from build123d import *

# Parameters (mm, degrees)
SKETCH1_R               = 14.287500000000001
BOSS_EXTRUDE1_DEPTH     = 165.1
CUT_EXTRUDE1_DEPTH      = 258.8795903614708
CUT_EXTRUDE1_DEPTH_BACK = 258.8795903614708
BOSS_EXTRUDE2_DEPTH     = 152.4
FILLET2_R               = 76.2


with BuildPart() as part:
    # Sketch1 → Boss-Extrude1 (new body)
    with BuildSketch(Plane.XY):
        with BuildLine():
            Line((6.759931115856893, 24.483940273347972), (-169.05197980207154, 73.02499999999999))
            ThreePointArc((-169.05197980207154, 73.02499999999999), (-184.15, 2.255e-14), (-169.05197980207154, -73.02499999999999))
            Line((-169.05197980207154, -73.02499999999999), (6.759931115856893, -24.483940273347972))
            ThreePointArc((6.759931115856893, -24.483940273347972), (25.40000000000002, 0), (6.759931115856893, 24.483940273347972))
        make_face()
        Circle(SKETCH1_R, mode=Mode.SUBTRACT)
    extrude(amount=-BOSS_EXTRUDE1_DEPTH)

    # Sketch2 → Cut-Extrude1 (cut, two sides: drawn at the far end of the back side and taken through both)
    with BuildSketch(Plane(origin=(0, 0, 0), x_dir=(1, 0, 0), z_dir=(0, 1, 0)).offset(-CUT_EXTRUDE1_DEPTH_BACK)):
        Polygon((-184.15, 158.75), (25.400000000000006, 158.75), (25.39999999999999, 6.35), (-184.14999999999998, 6.349999999999994), align=None)
    extrude(amount=CUT_EXTRUDE1_DEPTH + CUT_EXTRUDE1_DEPTH_BACK, mode=Mode.SUBTRACT)


with BuildPart() as cut_extrude1_piece_1:
    # of the separate pieces the step leaves, piece 1, a body of its own (cut_extrude1_pieces)
    add(part.part.solids().sort_by_distance((-169.051979802, -73.025, 0))[0])



with BuildPart() as cut_extrude1_piece_2:
    # of the separate pieces the step leaves, piece 2, a body of its own (cut_extrude1_pieces)
    add(part.part.solids().sort_by_distance((-169.051979802, -73.025, -158.75))[0])


with BuildPart() as cut_extrude1_piece_1_1:
    add(cut_extrude1_piece_1.part)

    add(cut_extrude1_piece_2.part)  # Boss-Extrude2 merges Cut-Extrude1 piece 2
    # Sketch3 → Boss-Extrude2 (add)
    with BuildSketch(Plane.XY.offset(-158.75)):
        with BuildLine():
            Line((-169.05197980207154, 73.02499999999999), (-164.155191747402, 71.67301377682864))
            ThreePointArc((-164.155191747402, 71.67301377682864), (-179.07, 3.242e-14), (-164.15519174740194, -71.67301377682858))
            Line((-164.15519174740194, -71.67301377682858), (-169.05197980207154, -73.02499999999998))
            ThreePointArc((-169.05197980207154, -73.02499999999998), (-184.15, 1.0433e-13), (-169.05197980207154, 73.02499999999999))
        make_face()
    extrude(amount=BOSS_EXTRUDE2_DEPTH)

    # Fillet2
    fillet2_edges = [cut_extrude1_piece_1_1.edges().sort_by_distance(p)[0] for p in [
        (-179.06999999999994, 1.066e-14, -6.349999999999994),
        (-179.06999999999994, 1.066e-14, -158.75),
    ]]
    fillet(fillet2_edges, radius=FILLET2_R - 0.0001)  # a hair under: the kernel refuses the full size


solid = cut_extrude1_piece_1_1.part
The listing builds one solid part. Answer for the finished solid, in the listing's coordinates (mm). Give positions to 0.01 mm unless a question says otherwise; leave off trailing zeros. Write each loop counter-clockwise with the first axis right and the second up, starting at its lowest first coordinate (ties: lowest second). Pieces come first, ordered by that corner, then holes. Notation, with made-up numbers: (30, 11.5) -> (70, 11.5) arc R18 ccw to (70, 33.5) -> close; hole circle Ø7 at (-2, 88). An arc over 180 degrees is marked (long way). One line per question, with ' | ' between items. Start each with the question number.
1. Section C-C (x = 0) is taken. Determine the outline of the cut face in (y, z).
2. Given pin 1 Ø8 at (y, z) = (53.5, -116.5) entering from -X; pin 2 Ø12 at (x, z) = (-129, -147) entering from +Y; pin 3 Ø5 at (x, z) = (-136.5, -19.5) entering from -Y, each flat-ended and moving along its own axis, determine where each tip first touches the part or whether it passes through.
3. Section B-B (y = 0) is taken. State how many separate pieces and enclosed holes the cut face has, plus the area to 3 significant figures.
4. Section A-A (x = -83.5) is taken. Determine the outline of the cut face in (y, z), plus the area to 3 significant figures.
5. For a pull along Z with two mould halves and no side action, classify faces 1 (the cylindrical face through (25.396, -0.463, -161.881)), 2 (the flat face through (-104, 1, 0)), 3 (the flat face through (-54, -1, -158.75)), 4 (the flat face through (-52, -1, -6.35)) as pulls with the +Z half, pulls with the -Z half, needs draft (parallel to the pull), parting line crosses it, or undercut.
6. Find the intervals of material crossed by probe 1 along Z at (x, y) = (-51, 13.5); probe 2 along Y at (x, z) = (0, -2); probe 3 along Z at (x, y) = (-145.5, -12), in increasing order.
Response values:
1) outline: (-26.35, -165.1) -> (-14.29, -165.1) -> (-14.29, -158.75) -> (-26.35, -158.75) -> close; (-26.35, -6.35) -> (-14.29, -6.35) -> (-14.29, 0) -> (-26.35, 0) -> close; (14.29, -165.1) -> (26.35, -165.1) -> (26.35, -158.75) -> (14.29, -158.75) -> close; (14.29, -6.35) -> (26.35, -6.35) -> (26.35, 0) -> (14.29, 0) -> close
2) pin 1: x = -177.37 | pin 2: y = 63.62 | pin 3: y = -64.73
3) separate pieces: 3 | enclosed holes: 0 | area: 5,560 mm2
4) outline: (-49.4, -165.1) -> (49.4, -165.1) -> (49.4, -158.75) -> (-49.4, -158.75) -> close; (-49.4, -6.35) -> (49.4, -6.35) -> (49.4, 0) -> (-49.4, 0) -> close | area: 1,250 mm2
5) face 1: needs draft | face 2: pulls with the +Z half | face 3: undercut | face 4: undercut
6) probe 1: -165.1 to -158.75, -6.35 to 0 | probe 2: -26.35 to -14.29, 14.29 to 26.35 | probe 3: -165.1 to -145.37, -19.73 to 0
